Autodesk Inventor part; units mm, degrees
ref_plane "YZ Plane" through (0, 0, 0) normal (1, 0, 0) x (0, 1, 0)
ref_plane "XZ Plane" through (0, 0, 0) normal (0, 1, 0) x (-1, 0, 0)
ref_plane "XY Plane" through (0, 0, 0) normal (0, 0, 1) x (1, 0, 0)
sketch "Sketch1" plane through (0, 0, 0) normal (0, 1, 0) x (-1, 0, 0)
  line L0 (-20.8041, 22.5) -> (20.8041, 22.5)
  line L1 (20.8041, 22.5) -> (20.8041, -22.5)
  line L2 (20.8041, -22.5) -> (-20.8041, -22.5)
  line L3 (-20.8041, -22.5) -> (-20.8041, 22.5)
  line L4 (-20.8041, 22.5) -> (20.8041, -22.5) construction
  line L5 (20.8041, 22.5) -> (-20.8041, -22.5) construction
  line L6 (-20.8041, -13.15) -> (20.8041, -13.15)
  line L7 (20.8041, -13.15) -> (20.8041, 13.15)
  line L8 (20.8041, 13.15) -> (-20.8041, 13.15)
  line L9 (-20.8041, 13.15) -> (-20.8041, -13.15)
  line L10 (-20.8041, -13.15) -> (20.8041, 13.15) construction
  line L11 (20.8041, -13.15) -> (-20.8041, 13.15) construction
  point P0 (0, 0)
  dimension "d0" = 26.3
  dimension "d1" = 45
extrude "Extrusion1" add sketch "Sketch1" along normal blind 3 contours L0 L1 L8 L3 | L6 L1 L2 L3
extrude "Extrusion2" add sketch "Sketch1" against normal blind 3
properties part number "ESPACIADOR_CREMALLERA" material "Steel, Mild, Welded"
Part model, mm, in its own coordinate system. A direction names the side the tool comes from. Coordinates: 2 decimals unless noted, no trailing zeros. Loops run counter-clockwise (first coordinate to the right, second up) from the corner with the lowest first, then second, coordinate; pieces in that order, holes last. Notation, with made-up numbers: (66, -32) - (86, -32) arc R29 cw to (86, -9) - close; hole circle Ø9 at (9.25, 30). An arc over 180 degrees is marked (long way). Write each question's results on one line, items separated by ' | '. Start each with the question number.
Q1. Slice it at B-B on x = -10.5. Give the cut face in (y, z).
Q2. Two-plate mould, pull along Z, no slides. Class faces 1 (the flat face through (0, 3, -18)), 2 (the flat face through (0, 0, -22.5)), 3 (the flat face through (0, 1, -13.15)): +Z half, -Z half, draft (parallel to the pull), parting line (faces both ways), or undercut.
Q3. Slice it at A-A on y = 0.75. Give the cut face in (x, z), and give its area (3 significant figures).
Q4. Slice it at C-C on z = 12.5. Give the cut face in (x, y), and give its area (3 significant figures).
Q5. Probe line 1 along Z through (x, y) = (2.5, 2.1); line 2 along Y through (x, z) = (9, 1). List the from-to ranges inside material, lowest first.
Q6. Which spindle directions (+Z, -Z, +X, -X, +Y, -Y) get a long thin tool onto all of the face, cutting with end or side? Do faces 4 (the flat face through (0, 0, 0)), 5 (the flat face through (20.804, -1, 0)). Say none if no direction does.
Answer:
1) outline: (-3, -22.5) - (3, -22.5) - (3, -13.15) - (0, -13.15) - (0, 13.15) - (3, 13.15) - (3, 22.5) - (-3, 22.5) - close
2) face 1: draft | face 2: -Z half | face 3: undercut
3) outline: (-20.8, -22.5) - (20.8, -22.5) - (20.8, -13.15) - (-20.8, -13.15) - close; (-20.8, 13.15) - (20.8, 13.15) - (20.8, 22.5) - (-20.8, 22.5) - close | area: 778 mm2
4) outline: (-20.8, -3) - (20.8, -3) - (20.8, 0) - (-20.8, 0) - close | area: 125 mm2
5) line 1: z = -22.5 to -13.15, 13.15 to 22.5 | line 2: y = -3 to 0
6) face 4: +X, -X, +Y | face 5: +Z, -Z, +X, +Y, -Y
